```python
from build123d import *

# Parameters (mm, degrees)
SKETCH_1_W          = 100
SKETCH_1_H          = 20
EXTRUDE_1_DEPTH     = 3
SKETCH_2_R          = 1.45
CUT_EXTRUDE_1_DEPTH = 6
SKETCH_3_W          = 100
SKETCH_3_H          = 3
CUT_EXTRUDE_2_DEPTH = 0.2
SKETCH_5_W          = 100
SKETCH_5_H          = 3
CUT_EXTRUDE_3_DEPTH = 0.2


with BuildPart() as part:
    # 草图1 → 凸台-拉伸1 (new body)
    with BuildSketch(Plane(origin=(0, 0, 0), x_dir=(1, 0, 0), z_dir=(0, 1, 0))):
        with Locations((-50, 10)):
            Rectangle(SKETCH_1_W, SKETCH_1_H)
    extrude(amount=EXTRUDE_1_DEPTH)

    # 草图2 → 切除-拉伸1 (cut)
    with BuildSketch(Plane(origin=(0, 3, 0), x_dir=(1, 0, 0), z_dir=(0, 1, 0))):
        with Locations(Location((-95, 15, 0), (0, 0, 270))):
            Circle(SKETCH_2_R)
        with Locations(Location((-95, 5, 0), (0, 0, 270))):
            Circle(SKETCH_2_R)
        with Locations(Location((-5, 5, 0), (0, 0, 270))):
            Circle(SKETCH_2_R)
        with Locations(Location((-5, 15, 0), (0, 0, 270))):
            Circle(SKETCH_2_R)
    extrude(amount=-CUT_EXTRUDE_1_DEPTH, mode=Mode.SUBTRACT)

    # 草图3 → 切除-拉伸2 (cut)
    with BuildSketch(Plane.XY):
        with Locations((-50, 1.5)):
            Rectangle(SKETCH_3_W, SKETCH_3_H)
    extrude(amount=-CUT_EXTRUDE_2_DEPTH, mode=Mode.SUBTRACT)

    # 草图5 → 切除-拉伸3 (cut)
    with BuildSketch(Plane(origin=(0, 0, -20), x_dir=(-1, 0, 0), z_dir=(0, 0, -1))):
        with Locations((50, 1.5)):
            Rectangle(SKETCH_5_W, SKETCH_5_H)
    extrude(amount=-CUT_EXTRUDE_3_DEPTH, mode=Mode.SUBTRACT)


solid = part.part
```
For this review, take the finished solid that the model builds, in its own axes (mm). Coordinates: 2 decimals unless noted, no trailing zeros. Order: outer loops, then holes, each group sorted by start corner. A loop starts at its lowest first (then second) coordinate and runs counter-clockwise, first axis right, second up. Notation, with made-up numbers: (23.5, 78.5) - (45.5, 78.5) arc R34 cw to (45.5, 114.5) - close; hole circle Ø9 at (77.5, -6). An arc over 180 degrees is marked (long way). Answer as a JSON object with one key per item and string values. Group by question number.
1. For probe 1 along Z at (x, y) = (-95, 0.9); probe 2 along X at (y, z) = (1.4, -15); probe 3 along Z at (x, y) = (-6, 2.45), list the stretches that pass through material, from the lowest coordinate up.
2. We need section A-A on x = -5. State the section outline as (y, z) points, then the cut area to 3 significant figures.
3. The part is to be moulded in two halves that separate along X. For faces 1 (the flat face through (-51, 3, -10)), 2 (the flat face through (-100, 1, -10)), 3 (the cylindrical face through (-93.562, 1.521, -5.189)), say which applies: pulls with the +X half, pulls with the -X half, needs draft (parallel to the pull), parting line crosses it, or undercut.
4. We need section B-B on z = -5. State the section outline as (x, y) points.
Final values:
{
 "1": {"probe 1": "-19.8 to -16.45, -13.55 to -6.45, -3.55 to -0.2", "probe 2": "-100 to -96.45, -93.55 to -6.45, -3.55 to 0", "probe 3": "-19.8 to -16.05, -13.95 to -6.05, -3.95 to -0.2"},
 "2": {"outline": "(0, -19.8) - (3, -19.8) - (3, -16.45) - (0, -16.45) - close; (0, -13.55) - (3, -13.55) - (3, -6.45) - (0, -6.45) - close; (0, -3.55) - (3, -3.55) - (3, -0.2) - (0, -0.2) - close", "area": "41.4 mm²"},
 "3": {"face 1": "needs draft", "face 2": "pulls with the -X half", "face 3": "undercut"},
 "4": {"outline": "(-100, 0) - (-96.45, 0) - (-96.45, 3) - (-100, 3) - close; (-93.55, 0) - (-6.45, 0) - (-6.45, 3) - (-93.55, 3) - close; (-3.55, 0) - (0, 0) - (0, 3) - (-3.55, 3) - close"}
}
